Verification items for the finished model (mm, model axes). A direction names the side the tool comes from. Coordinates: 2 decimals unless noted, no trailing zeros.
Q1. Material ranges on probe 1 along X at (y, z) = (207, -4); probe 2 along Z at (x, y) = (-67.5, 221); probe 3 along Z at (x, y) = (-9.5, 206.5), recorded low to high.
Q2. Access from +Z, -Z, +X, -X, +Y, -Y to the whole of each face (thin tool, end or side, straight path). Record for faces 1 (the face through (-86.65, 216.24, -89.88)), 2 (the face through (-130.48, 208.09, 17.18)), 3 (the face through (17.18, 208.09, -130.48)).
Q3. Mould release check, pull along X, two halves, no side actions. Record for faces 4 (the face through (-105.207, 215.744, 60.741)), 5 (the face through (-102.72, 203.76, -99.02)), 6 (the face through (-74.635, 220.486, -77.422)): +X half, -X half, draft (parallel to the pull), parting line (faces both ways), or undercut.
Q4. Go/stop test with flat-tipped pins: P1, Ø6, axis at x = -10, y = 226.5, coming from the -Z side; P2, Ø10, axis at x = 22, y = 218, coming from the -Z side; P3, Ø6, axis at x = -101.5, z = -70.5, coming from the -Y side. Record where each tip stops, or that it passes through.
```python
from build123d import *
from build123d.topology import SkipClean

# Parameters (mm, degrees)
REVOLVE1_ANGLE           = 30
REVOLVE1_OTHER_WAY_ANGLE = 120
REVOLVE2_ANGLE           = 15
CIRPATTERN1_COUNT        = 4
REVOLVE4_ANGLE           = 16
CUT_REVOLVE4_START       = -250
CUT_REVOLVE4_OUTLINE_R   = 4
CUT_REVOLVE4_DEPTH       = 1.5
CUT_REVOLVE4_START_2     = -248.5
CUT_REVOLVE4_2_OUTLINE_R = 1
CUT_REVOLVE4_2_DEPTH     = 1.00202
FILLET2_R                = 5
CIRPATTERN5_COUNT        = 2
CIRPATTERN5_ANGLE        = 90
FILLET2_OF_CIRPATTERN5_R = 5


# Read off the part's stored shape, not the designer's step: Revolve2, Revolve4, Cut-Revolve4
with BuildPart() as part:
    # Sketch1 → Revolve1 (revolve)
    with BuildSketch(Plane.XY):
        with BuildLine():
            ThreePointArc((-142.533744, 203.559283), (-133.518953, 209.582774), (-124.25, 215.207313))
            Line((-124.25, 215.207313), (-125, 216.506351))
            ThreePointArc((-125, 216.506351), (-134.324902, 210.847861), (-143.394109, 204.788011))
            Line((-143.394109, 204.788011), (-142.533744, 203.559283))
        make_face()
        with BuildLine():
            ThreePointArc((-124.25, 215.207313), (-64.316533, 240.032568), (0, 248.5))
            Line((0, 248.5), (0, 250))
            ThreePointArc((0, 250), (-64.704761, 241.481457), (-125, 216.506351))
            Line((-125, 216.506351), (-124.25, 215.207313))
        make_face()
        with BuildLine():
            ThreePointArc((-122.5, 212.176224), (-63.410666, 236.651827), (0, 245))
            Line((0, 245), (0, 248.5))
            ThreePointArc((0, 248.5), (-64.316533, 240.032568), (-124.25, 215.207313))
            Line((-124.25, 215.207313), (-122.5, 212.176224))
        make_face()
    revolve(axis=Axis((0, 0, 0), (0, 1, 0)), revolution_arc=REVOLVE1_ANGLE)

    # Sketch1 → Revolve1 other way (revolve)
    with SkipClean():  # the faces are left unmerged after this step: merging them gives an invalid solid
        with BuildSketch(Plane.XY):
            with BuildLine():
                ThreePointArc((-142.533744, 203.559283), (-133.518953, 209.582774), (-124.25, 215.207313))
                Line((-124.25, 215.207313), (-125, 216.506351))
                ThreePointArc((-125, 216.506351), (-134.324902, 210.847861), (-143.394109, 204.788011))
                Line((-143.394109, 204.788011), (-142.533744, 203.559283))
            make_face()
            with BuildLine():
                ThreePointArc((-124.25, 215.207313), (-64.316533, 240.032568), (0, 248.5))
                Line((0, 248.5), (0, 250))
                ThreePointArc((0, 250), (-64.704761, 241.481457), (-125, 216.506351))
                Line((-125, 216.506351), (-124.25, 215.207313))
            make_face()
            with BuildLine():
                ThreePointArc((-122.5, 212.176224), (-63.410666, 236.651827), (0, 245))
                Line((0, 245), (0, 248.5))
                ThreePointArc((0, 248.5), (-64.316533, 240.032568), (-124.25, 215.207313))
                Line((-124.25, 215.207313), (-122.5, 212.176224))
            make_face()
        revolve(axis=Axis((0, 0, 0), (0, -1, 0)), revolution_arc=REVOLVE1_OTHER_WAY_ANGLE)

    # Revolve2 outline → Revolve2 (revolve)
    with SkipClean():  # the faces are left unmerged after this step: merging them gives an invalid solid
        with BuildSketch(Plane(origin=(0, 0, 0), x_dir=(-0.9914448613738103, 0, -0.13052619222005243), z_dir=(0.13052619222005243, 0, -0.9914448613738103))):
            with BuildLine():
                Line((133.4007, 205.497575), (135.306424, 208.433255))
                Line((135.306424, 208.433255), (135.306424, 209.582774))
                Line((135.306424, 209.582774), (133.518953, 209.582774))
                Line((133.518953, 209.582774), (132.713003, 208.317687))
                ThreePointArc((132.713003, 208.317687), (130.890058, 209.46788), (129.057145, 210.602121))
                Line((129.057145, 210.602121), (128.012148, 208.89684))
                ThreePointArc((128.012148, 208.89684), (130.717474, 207.214724), (133.4007, 205.497575))
            make_face()
        revolve2 = revolve(axis=Axis((0, 0, 0), (0, 1, 0)), revolution_arc=REVOLVE2_ANGLE)

    # CirPattern1: Revolve2 ×4 about axis, 2 skipped
    with SkipClean():  # the faces are left unmerged after this step: merging them gives an invalid solid
        cirpattern1_axis = Axis((0, 0, 0), (0, -1, 0))
        add([revolve2.rotate(cirpattern1_axis, i * 360 / CIRPATTERN1_COUNT) for i in range(1, CIRPATTERN1_COUNT) if i not in (2, 3)])

    # Sketch4 → Cut-Revolve1 (revolve, cut)
    with BuildSketch(Plane.XY):
        with BuildLine():
            Line((0, 250), (0, 0))
            Line((0, 0), (109.592787, 224.698512))
            ThreePointArc((109.592787, 224.698512), (56.237764, 243.592516), (0, 250))
        make_face()
    revolve(axis=Axis((0, 0, 0), (0, 1, 0)), mode=Mode.SUBTRACT)

    # Revolve4 outline → Revolve4 (revolve)
    with BuildSketch(Plane(origin=(0, 0, 0), x_dir=(-0.9902680687415703, 0, -0.13917310096006574), z_dir=(0.13917310096006574, 0, -0.9902680687415703))):
        with BuildLine():
            Line((108.496859, 222.451526), (114.084698, 222.451526))
            ThreePointArc((114.084698, 222.451526), (89.899679, 233.276762), (64.704761, 241.481457))
            Line((64.704761, 241.481457), (64.057714, 239.066642))
            ThreePointArc((64.057714, 239.066642), (86.676327, 231.826367), (108.496859, 222.451526))
        make_face()
    revolve4 = revolve(axis=Axis((0, 0, 0), (0, 1, 0)), revolution_arc=REVOLVE4_ANGLE)

    # Cut-Revolve4 outline → Cut-Revolve4 (cut)
    with BuildSketch(Plane(origin=(0, 0, 0), x_dir=(0.956304755963035, 0.29237170472273805, 0), z_dir=(0.29237170472273805, -0.9563047559630351, 0)).offset(CUT_REVOLVE4_START)):
        Circle(CUT_REVOLVE4_OUTLINE_R)
    cut_revolve4 = extrude(amount=CUT_REVOLVE4_DEPTH, mode=Mode.SUBTRACT)

    # Cut-Revolve4 2 outline → Cut-Revolve4 2 (cut)
    with BuildSketch(Plane(origin=(0, 0, 0), x_dir=(0.956304755963035, 0.29237170472273805, 0), z_dir=(0.29237170472273805, -0.9563047559630351, 0)).offset(CUT_REVOLVE4_START_2)):
        Circle(CUT_REVOLVE4_2_OUTLINE_R)
    cut_revolve4_2 = extrude(amount=CUT_REVOLVE4_2_DEPTH, mode=Mode.SUBTRACT)

    # Fillet2
    fillet2_edges = [part.edges().sort_by_distance(p)[0] for p in [
        (-63.754684, 240.274049, -8.960136),
        (-63.754684, 240.274049, 8.960136),
    ]]
    fillet(fillet2_edges, radius=FILLET2_R)

    # CirPattern5: Revolve4, Cut-Revolve4, Cut-Revolve4 2 ×2 about axis
    cirpattern5_axis = Axis((0, 0, 0), (0, -1, 0))
    add([revolve4.rotate(cirpattern5_axis, i * CIRPATTERN5_ANGLE / (CIRPATTERN5_COUNT - 1)) for i in range(1, CIRPATTERN5_COUNT)])
    add([cut_revolve4.rotate(cirpattern5_axis, i * CIRPATTERN5_ANGLE / (CIRPATTERN5_COUNT - 1)) for i in range(1, CIRPATTERN5_COUNT)], mode=Mode.SUBTRACT)
    add([cut_revolve4_2.rotate(cirpattern5_axis, i * CIRPATTERN5_ANGLE / (CIRPATTERN5_COUNT - 1)) for i in range(1, CIRPATTERN5_COUNT)], mode=Mode.SUBTRACT)

    # Fillet2 of CirPattern5
    fillet2_of_cirpattern5_edges = [part.edges().sort_by_distance(p)[0] for p in [
        (8.960136, 240.274049, -63.754684),
        (-8.960136, 240.274049, -63.754684),
    ]]
    fillet(fillet2_of_cirpattern5_edges, radius=FILLET2_OF_CIRPATTERN5_R)

    # Sketch11 → Cut-Revolve5 (revolve, cut)
    with BuildSketch(Plane.XY):
        with BuildLine():
            ThreePointArc((-125.615023, 215.571603), (-125.182763, 215.822904), (-124.75, 216.073338))
            Line((-124.75, 216.073338), (-125, 216.506351))
            ThreePointArc((-125, 216.506351), (-125.432764, 216.255917), (-125.865025, 216.004619))
            Line((-125.865025, 216.004619), (-125.615023, 215.571603))
        make_face()
    revolve(axis=Axis((0, 0, 0), (0, 1, 0)), mode=Mode.SUBTRACT)


solid = part.part
```
Geometry check:
1. probe 1: x = -140.12 to -137.43, -134.32 to -131
1. probe 2: z = -95.41 to -84.04
1. probe 3: z = -140.6 to -137.91, -133.71 to -131.5
2. face 1: none
2. face 2: +X, -Y
2. face 3: +Z, -Y
3. face 4: +X half
3. face 5: parting line
3. face 6: undercut
4. P1: stops at z = -111.58
4. P2: stops at z = -129.07
4. P3: stops at y = 212.18
